```python
from build123d import *

# Parameters (mm, degrees)
EXTRUDE_1_DEPTH     = 15
CHAMFER_1_SIZE      = 1
CHAMFER_2_SIZE      = 1.5
SKETCH_2_R          = 6
CUT_EXTRUDE_1_DEPTH = 7
SKETCH_3_R          = 3.5
CUT_EXTRUDE_2_DEPTH = 4.5
SKETCH_4_R          = 1
CUT_EXTRUDE_3_DEPTH = 1.5
CHAMFER_5_SIZE      = 1


with BuildPart() as part:
    # Эскиз1 → Бобышка-Вытянуть1 (new body)
    with BuildSketch(Plane(origin=(0, 0, 0), x_dir=(1, 0, 0), z_dir=(0, 1, 0))):
        Polygon((-2.899494937, 7), (-7, 2.899494937), (-7, -2.899494937), (-2.899494937, -7), (2.899494937, -7), (7, -2.899494937), (7, 2.899494937), (2.899494937, 7), align=None)
    extrude(amount=EXTRUDE_1_DEPTH)

    # Фаска1
    chamfer_1_edges = [part.edges().sort_by_distance(p)[0] for p in [
        (-4.949747468, 15, -4.949747468),
        (-7, 15, 0),
        (-4.949747468, 15, 4.949747468),
        (0, 15, 7),
        (4.949747468, 15, 4.949747468),
        (7, 15, 0),
        (4.949747468, 15, -4.949747468),
        (0, 15, -7),
    ]]
    chamfer(chamfer_1_edges, length=CHAMFER_1_SIZE)

    # Фаска2
    chamfer_2_edges = [part.edges().sort_by_distance(p)[0] for p in [
        (-4.949747468, 0, 4.949747468),
        (-7, 0, 0),
        (-4.949747468, 0, -4.949747468),
        (0, 0, -7),
        (4.949747468, 0, -4.949747468),
        (7, 0, 0),
        (4.949747468, 0, 4.949747468),
        (0, 0, 7),
    ]]
    chamfer(chamfer_2_edges, length=CHAMFER_2_SIZE)

    # Эскиз2 → Вырез-Вытянуть1 (cut)
    with BuildSketch(Plane(origin=(0, 15, 0), x_dir=(1, 0, 0), z_dir=(0, 1, 0))):
        with Locations(Location((0, 0, 0), (0, 0, 270))):
            Circle(SKETCH_2_R)
    extrude(amount=-CUT_EXTRUDE_1_DEPTH, mode=Mode.SUBTRACT)

    # Эскиз3 → Вырез-Вытянуть2 (cut)
    with BuildSketch(Plane.XZ):
        with Locations(Location((0, 0, 0), (0, 0, 270))):
            Circle(SKETCH_3_R)
    extrude(amount=-CUT_EXTRUDE_2_DEPTH, mode=Mode.SUBTRACT)

    # Эскиз4 → Вырез-Вытянуть3 (cut)
    with BuildSketch(Plane.XZ.offset(-4.5)):
        with Locations(Location((0, 0, 0), (0, 0, 270))):
            Circle(SKETCH_4_R)
    extrude(amount=-CUT_EXTRUDE_3_DEPTH, mode=Mode.SUBTRACT)

    # Фаска5
    chamfer_5_edges = [part.edges().sort_by_distance(p)[0] for p in [
        (0, 6, 1),
    ]]
    chamfer(chamfer_5_edges, length=CHAMFER_5_SIZE)


solid = part.part
```
CAD build for the part. Positions are in the model's coordinates, mm. Round coordinates to 2 decimals unless told otherwise and drop trailing zeros. Write each loop counter-clockwise with the first axis right and the second up, starting at its lowest first coordinate (ties: lowest second). Pieces come first, ordered by that corner, then holes.
Item 1: Drop flat-ended pins along their axis: pin 1 Ø8 at (x, z) = (-1, 0.5) entering from +Y; pin 2 Ø3 at (y, z) = (5.5, 4.5) entering from +X; pin 3 Ø6.5 at (x, z) = (0, 0) entering from -Y. Give the stop position or say it passes through.
Filled in:
pin 1: stops at y = 8
pin 2: stops at x = 6.9
pin 3: stops at y = 4.5
Item 2: Band-saw the part on B-B on z = -2. Write the cut outline in (x, y).
Filled in:
outline: (-7, 1.5) - (-5.5, 0) - (-2.87, 0) - (-2.87, 4.5) - (2.87, 4.5) - (2.87, 0) - (5.5, 0) - (7, 1.5) - (7, 14) - (6, 15) - (5.66, 15) - (5.66, 8) - (-5.66, 8) - (-5.66, 15) - (-6, 15) - (-7, 14) - close
Item 3: Mould opens along Z. For faces 1 (the flat face through (0, 14.5, -6.5)), 2 (the flat face through (0, 8, 0)), 3 (the flat face through (2.4, 15, 5.7)), 4 (the flat face through (0, 14.5, 6.5)) say: released by +Z, released by -Z, zero draft, split by the parting line, or undercut.
Filled in:
face 1: released by -Z
face 2: undercut
face 3: zero draft
face 4: released by +Z
Item 4: Band-saw the part on A-A on y = 8.75. Write the cut outline in (x, z).
Filled in:
outline: (-7, -2.9) - (-2.9, -7) - (2.9, -7) - (7, -2.9) - (7, 2.9) - (2.9, 7) - (-2.9, 7) - (-7, 2.9) - close; hole circle Ø12 at (0, 0)
Item 5: Band-saw the part on C-C on y = 4.25. Write the cut outline in (x, z), then the cut area to 3 significant figures.
Filled in:
outline: (-7, -2.9) - (-2.9, -7) - (2.9, -7) - (7, -2.9) - (7, 2.9) - (2.9, 7) - (-2.9, 7) - (-7, 2.9) - close; hole circle Ø7 at (0, 0)
area: 124 mm2
Item 6: Drill centre lines: L1, parallel to X at y = 2.65, z = 0; L2, parallel to X at y = 10.5, z = 0; L3, parallel to Y at x = -2.5, z = 1. Where is each one in solid material? Low to high.
Filled in:
L1: x = -7 to -3.5, 3.5 to 7
L2: x = -7 to -6, 6 to 7
L3: y = 4.5 to 8
